Check sheet for the modelled part. Datum: model origin and axes. Units: mm. Give positions to 0.01 mm unless a question says otherwise; leave off trailing zeros. Write each loop counter-clockwise with the first axis right and the second up, starting at its lowest first coordinate (ties: lowest second). Pieces come first, ordered by that corner, then holes. Notation, with made-up numbers: (41, -6.5) -> (54, -6.5) arc R21 cw to (54, 6.5) -> close; hole circle Ø7 at (87.25, 19). An arc over 180 degrees is marked (long way). Write each question's results on one line, items separated by ' | '. Start each with the question number.
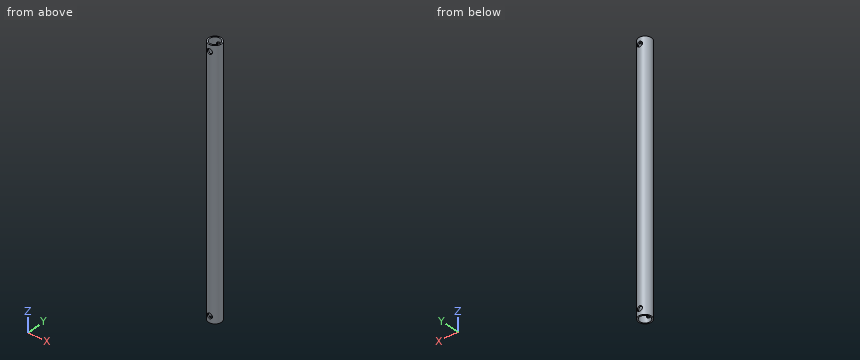
```python
from build123d import *

# Parameters (mm, degrees)
SKETCH_1_R               = 10
SKETCH_1_R_2             = 8
EXTRUDE_1_DEPTH          = 400
SKETCH_2_R               = 4
CUT_EXTRUDE_1_DEPTH      = 11
CUT_EXTRUDE_1_DEPTH_BACK = 11


with BuildPart() as part:
    # 草图1 → 凸台-拉伸1 (new body)
    with BuildSketch(Plane.XY):
        Circle(SKETCH_1_R)
        Circle(SKETCH_1_R_2, mode=Mode.SUBTRACT)
    extrude(amount=EXTRUDE_1_DEPTH)

    # 草图2 → 切除-拉伸1 (cut, two sides)
    with BuildSketch(Plane(origin=(0, 0, 0), x_dir=(1, 0, 0), z_dir=(0, 1, 0))) as cut_extrude_1_sk:
        with Locations((0, -10)):
            Circle(SKETCH_2_R)
        with Locations((0, -390)):
            Circle(SKETCH_2_R)
    extrude(amount=CUT_EXTRUDE_1_DEPTH, mode=Mode.SUBTRACT)
    extrude(cut_extrude_1_sk.sketch, amount=-CUT_EXTRUDE_1_DEPTH_BACK, mode=Mode.SUBTRACT)


solid = part.part
```
Item 1: Section check B-B on x = 0. Record the boundary of the cut face in (y, z).
Item 2: Section check A-A on y = 0. Record the boundary of the cut face in (x, z), then the cut area to 3 significant figures.
Item 3: Depth check by flat-ended pin: pin 1 Ø6 at (x, z) = (-1, 229.5) entering from +Y; pin 2 Ø1 at (y, z) = (4, 302.5) entering from +X; pin 3 Ø5 at (x, z) = (-3.5, 44.5) entering from -Y; pin 4 Ø8 at (y, z) = (-5.5, 166) entering from -X. Enter the tip coordinate at first touch or a pass-through.
Item 4: Thickness scan on probe 1 along Z at (x, y) = (0, -8.6); probe 2 along Y at (x, z) = (0, 235); probe 3 along X at (y, z) = (1.25, 178.5). Record the ranges inside material, lowest first. Write a range as from..to.
Item 5: Section check C-C on z = 390. Record the boundary of the cut face in (x, y).
Item 6: Section check D-D on z = 65.5. Record the boundary of the cut face in (x, y).
Check sheet entries:
1) outline: (-10, 0) -> (-8, 0) -> (-8, 6) -> (-10, 6) -> close; (-10, 14) -> (-8, 14) -> (-8, 386) -> (-10, 386) -> close; (-10, 394) -> (-8, 394) -> (-8, 400) -> (-10, 400) -> close; (8, 0) -> (10, 0) -> (10, 6) -> (8, 6) -> close; (8, 14) -> (10, 14) -> (10, 386) -> (8, 386) -> close; (8, 394) -> (10, 394) -> (10, 400) -> (8, 400) -> close
2) outline: (-10, 0) -> (-8, 0) -> (-8, 400) -> (-10, 400) -> close; (8, 0) -> (10, 0) -> (10, 400) -> (8, 400) -> close | area: 1,600 mm^2
3) pin 1: stops at y = 10 | pin 2: stops at x = 9.37 | pin 3: stops at y = -9.95 | pin 4: stops at x = -9.89
4) probe 1: z = 0..6, 14..386, 394..400 | probe 2: y = -10..-8, 8..10 | probe 3: x = -9.92..-7.9, 7.9..9.92
5) outline: (-4, -9.17) -> (-4, -6.93) arc R8 cw to (-4, 6.93) -> (-4, 9.17) arc R10 ccw to start; (4, -9.17) arc R10 ccw to (4, 9.17) -> (4, 6.93) arc R8 cw to (4, -6.93) -> close
6) outline: circle Ø20 at (0, 0); hole circle Ø16 at (0, 0)
